from build123d import *

# Parameters (mm, degrees)
F0_R     = 65
F0_R_2   = 55
F1_DEPTH = 20
F3_DEPTH = 20
F4_R     = 4.5
F5_DEPTH = 172.996652


with BuildPart() as f1:
    # F0 (on Top) → F1 (new body)
    with BuildSketch(Plane.XY):
        Circle(F0_R)
        Circle(F0_R_2, mode=Mode.SUBTRACT)
    extrude(amount=F1_DEPTH)

    # F2 (on Front) → F3 (join)
    with BuildSketch(Plane.XZ):
        Polygon((-70.995652, 0), (-55.995652, 0), (-55.995652, 90), (-70.995652, 90), (-107.995652, 90), (-107.995652, 30), (-92.995652, 30), (-92.995652, 75), (-70.995652, 75), align=None)
    extrude(amount=F3_DEPTH)

    # F4 (on face) → F5 (cut, through all)
    with BuildSketch(Plane(origin=(-107.995652, 0, 0), x_dir=(0, -1, 0), z_dir=(-1, 0, 0))):
        with Locations((11, 48.7937)):
            Circle(F4_R)
    extrude(amount=-F5_DEPTH, mode=Mode.SUBTRACT)


solid = f1.part
Verification items for the finished model (mm, model axes). A direction names the side the tool comes from. Coordinates: 2 decimals unless noted, no trailing zeros. Loops run counter-clockwise (first coordinate to the right, second up) from the corner with the lowest first, then second, coordinate; pieces in that order, holes last. Notation, with made-up numbers: (65.5, 34) -> (112.5, 34) arc R19 ccw to (112.5, 63) -> close; hole circle Ø8 at (-6, -22.5). An arc over 180 degrees is marked (long way). Write each question's results on one line, items separated by ' | '.
Item 1: Tool access check on faces 4 (the face through (-70.996, -10, 38)), 5 (the face through (-100.6, -13.4, 52.6)), 6 (the face through (-55.996, -10, 55)), 7 (the face through (-101, -10, 30)). Record the directions out of +Z, -Z, +X, -X, +Y, -Y that give a thin tool (end or side, any length) a straight path to the whole face; none if there is none.
Found:
face 4: -Z, +Y, -Y | face 5: +X, -X | face 6: +Z, +X, +Y, -Y | face 7: -Z, -X, +Y, -Y
Item 2: Section check A-A, the plane z = 64. Enter the section's corners in (x, y).
Found:
outline: (-108, -20) -> (-93, -20) -> (-93, 0) -> (-108, 0) -> close; (-71, -20) -> (-56, -20) -> (-56, 0) -> (-71, 0) -> close
Item 3: Mould release check, pull along Z, two halves, no side actions. Record for faces 1 (the face through (-82, -10, 75)), 2 (the face through (-92.996, -7.6, 52.2)), 3 (the face through (-63.6, -13.4, 52.6)): +Z half, -Z half, draft (parallel to the pull), parting line (faces both ways), or undercut.
Found:
face 1: -Z half | face 2: draft | face 3: undercut
Item 4: Section check D-D, the plane z = 15.5. Enter the section's corners in (x, y).
Found:
outline: (-71, -20) -> (-61.85, -20) arc R65 ccw (long way) to (-65, 0) -> (-71, 0) -> close; hole circle Ø110 at (0, 0)
Item 5: Gauge pin test, flat ends, axial feed: pin 1 (6 mm diameter, centred on y = -6, z = 39.5, fed in from +X); pin 2 (1.5 mm diameter, centred on x = -42.5, y = 47, fed in from +Z); pin 3 (12 mm diameter, centred on x = -99.5, y = -8, fed in from -Z); pin 4 (16 mm diameter, centred on y = -14, z = 47, fed in from -X). Record the tip position at first contact, or that the pin passes through.
Found:
pin 1: stops at x = -56 | pin 2: stops at z = 20 | pin 3: stops at z = 30 | pin 4: stops at x = -108
Item 6: Section check C-C, the plane y = -11. Enter the section's corners in (x, z), plus the area to 3 significant figures.
Found:
outline: (-108, 30) -> (-93, 30) -> (-93, 44.29) -> (-108, 44.29) -> close; (-108, 53.29) -> (-93, 53.29) -> (-93, 75) -> (-71, 75) -> (-71, 53.29) -> (-56, 53.29) -> (-56, 90) -> (-108, 90) -> close; (-71, 0) -> (-53.89, 0) -> (-53.89, 20) -> (-56, 20) -> (-56, 44.29) -> (-71, 44.29) -> close; (53.89, 0) -> (64.06, 0) -> (64.06, 20) -> (53.89, 20) -> close | area: 2,560 mm2
Item 7: Section check B-B, the plane x = 0. Enter the section's corners in (y, z), plus the area to 3 significant figures.
Found:
outline: (-65, 0) -> (-55, 0) -> (-55, 20) -> (-65, 20) -> close; (55, 0) -> (65, 0) -> (65, 20) -> (55, 20) -> close | area: 400 mm2
Item 8: Material ranges on L1, parallel to Z at x = -61, y = -11; L2, parallel to Y at x = 0, z = 11.5; L3, parallel to Z at x = -97, y = -11, recorded low to high.
Found:
L1: z = 0 to 44.29, 53.29 to 90 | L2: y = -65 to -55, 55 to 65 | L3: z = 30 to 44.29, 53.29 to 90
